Autodesk Inventor part; units mm, degrees
ref_plane "YZ Plane" through (0, 0, 0) normal (1, 0, 0) x (0, 1, 0)
ref_plane "XZ Plane" through (0, 0, 0) normal (0, 1, 0) x (-1, 0, 0)
ref_plane "XY Plane" through (0, 0, 0) normal (0, 0, 1) x (1, 0, 0)
sketch "スケッチ1" plane through (0, 0, 0) normal (0, 0, 1) x (1, 0, 0)
  circle A0 centre (0, 0) radius 1.5
  dimension "d0" = 3
extrude "押し出し1" add sketch "スケッチ1" along normal blind 6
sketch "スケッチ2" plane through (0, 0, 6) normal (0, 0, 1) x (1, 0, 0)
  circle A0 centre (0, 0) radius 1.5
  circle A1 centre (0, 0) radius 3
  dimension "d3" = 6
extrude "押し出し2" add sketch "スケッチ2" along normal blind 1.75 contours A0 | A1
thread "ねじ1"
chamfer "面取り1" distance 1.5 angle 45 1 edges at (-3, 0, 6)
sketch "スケッチ4" plane through (0, 0, 0) normal (0, 0, -1) x (-1, 0, 0)
  circle A0 centre (0, 0) radius 1.5
extrude "押し出し4" add sketch "スケッチ4" along normal blind 4
sketch "スケッチ5" plane through (0, 0, -4) normal (0, 0, -1) x (-1, 0, 0)
  circle A0 centre (0, 0) radius 1.5
extrude "押し出し5" cut sketch "スケッチ5" against normal blind 2
sketch "スケッチ6" plane through (0, 0, -2) normal (0, 0, -1) x (-1, 0, 0)
  circle A0 centre (0, 0) radius 1.5
extrude "押し出し6" add sketch "スケッチ6" along normal blind 25.25
properties part number "SB　35mm皿ネジ" material "Steel, Mild"
Source: CAD feature listing. Evaluate the final solid. Frame: model axes, mm. Coordinates: 2 decimals unless noted, no trailing zeros. Order: outer loops, then holes, each group sorted by start corner. A loop starts at its lowest first (then second) coordinate and runs counter-clockwise, first axis right, second up. Notation, with made-up numbers: M -31,7 L 16,7 A28 cw 16,30 Z; hole C -15.5,39 d9. An arc over 180 degrees is marked long. Write each question's results on one line, items separated by ' | '. Start each with the question number.
1) Section query C-C (z = -12.5). Return the cut outline in (x, y).
2) Line query: line 1 (Y direction, x = 0, z = -25); line 2 (X direction, y = -0.6, z = -14); line 3 (Y direction, x = -0.45, z = -16). Output: solid intervals per line, ascending. Write a range as from..to.
3) Contact query for a flat-ended pin moving along its axis: pin 1 Ø3 at (x, z) = (-0.5, 0) entering from -Y. Output: stop coordinate, or through.
Answers:
1) outline: C 0,0 d3
2) line 1: y = -1.5..1.5 | line 2: x = -1.37..1.37 | line 3: y = -1.43..1.43
3) pin 1: stops at y = -1.5
